Verification items for the finished model (mm, model axes). A direction names the side the tool comes from. Coordinates: 2 decimals unless noted, no trailing zeros. Write each loop counter-clockwise with the first axis right and the second up, starting at its lowest first coordinate (ties: lowest second). Pieces come first, ordered by that corner, then holes. Notation, with made-up numbers: (55, -32) -> (69, -32) arc R14 cw to (69, -20) -> close; hole circle Ø11 at (41.5, 56.25). An arc over 180 degrees is marked (long way). Write each question's results on one line, items separated by ' | '. Start each with the question number.
from build123d import *

# Parameters (mm, degrees)
F0_W     = 121.512517333
F0_H     = 63.0381852388
F1_DEPTH = 2.54
F3_R     = 10.4902
F2_R     = 10.4902
F2_R_2   = 10.4891359602
F4_DEPTH = 5.08
F5_W     = 24.793356657
F5_H     = 18.3770691669
F6_DEPTH = 4.4237


with BuildPart() as f1:
    # F0 (on Top) → F1 (new body)
    with BuildSketch(Plane.XY):
        Rectangle(F0_W, F0_H)
    extrude(amount=F1_DEPTH)

    # F3 (on face) + F2 (on face) → F4 (join)
    with BuildSketch(Plane(origin=(0, 31.5190926194, 0), x_dir=(-1, 0, 0), z_dir=(0, 1, 0))):
        with Locations((-47.3014861345, 0)):
            Circle(F3_R)
        with Locations((39.0958227217, 0)):
            Circle(F3_R)
    with BuildSketch(Plane.XZ.offset(31.5190926194)):
        with Locations((-42.2156155109, 0)):
            Circle(F2_R)
        with Locations((44.4975420833, 0)):
            Circle(F2_R_2)
    extrude(amount=F4_DEPTH, dir=(0, 1, 0))

    # F5 (on face) → F6 (join)
    with BuildSketch(Plane.YZ.offset(60.7562586665)):
        with Locations((-0.8818171918, 11.7285345834)):
            Rectangle(F5_W, F5_H)
    extrude(amount=-F6_DEPTH)


solid = f1.part
1. Material ranges on probe 1 along Y at (x, z) = (-40, -9); probe 2 along Z at (x, y) = (14.5, 8); probe 3 along Y at (x, z) = (28, 1.5), recorded low to high. Write a range as from..to.
2. Sectioned sample at B-B on z = -8. Record the cut outline in (x, y), plus the area to 3 significant figures.
3. Depth check by flat-ended pin: pin 1 Ø3 at (x, y) = (-18.5, -15) entering from -Z; pin 2 Ø5.5 at (y, z) = (2, 11.5) entering from -X; pin 3 Ø3.5 at (x, z) = (59.5, 15) entering from -Y. Enter the tip coordinate at first touch or a pass-through.
4. Mould release check, pull along Y, two halves, no side actions. Record for faces 5 (the flat face through (-39, 36.599, 0)), 6 (the cylindrical face through (-42.446, -29.015, -10.488)), 7 (the flat face through (47, 31.519, -4)): +Y half, -Y half, draft (parallel to the pull), parting line (faces both ways), or undercut.
5. Sectioned sample at D-D on z = 17. Record the cut outline in (x, y), plus the area to 3 significant figures.
6. Sectioned sample at C-C on x = -45.5. Record the cut outline in (y, z).
7. Tool access check on faces 1 (the cylindrical face through (-42.02, -29.01, 10.49)), 2 (the cylindrical face through (-28.616, 34.024, 0.461)), 3 (the flat face through (-39, 31.519, -4)), 4 (the flat face through (-42, -26.439, 6)). Record the directions out of +Z, -Z, +X, -X, +Y, -Y that give a thin tool (end or side, any length) a straight path to the whole face; none if there is none.
8. Sectioned sample at A-A on y = -3. Record the cut outline in (x, z), plus the area to 3 significant figures.
Computed values:
1) probe 1: y = -31.52..-26.44, 31.52..36.6 | probe 2: z = 0..2.54 | probe 3: y = -31.52..31.52
2) outline: (-49, -31.52) -> (-35.43, -31.52) -> (-35.43, -26.44) -> (-49, -26.44) -> close; (-45.88, 31.52) -> (-32.31, 31.52) -> (-32.31, 36.6) -> (-45.88, 36.6) -> close; (37.71, -31.52) -> (51.28, -31.52) -> (51.28, -26.44) -> (37.71, -26.44) -> close; (40.52, 31.52) -> (54.09, 31.52) -> (54.09, 36.6) -> (40.52, 36.6) -> close | area: 276 mm^2
3) pin 1: stops at z = 0 | pin 2: stops at x = 56.33 | pin 3: stops at y = -13.28
4) face 5: +Y half | face 6: draft | face 7: undercut
5) outline: (56.33, -13.28) -> (60.76, -13.28) -> (60.76, 11.51) -> (56.33, 11.51) -> close | area: 110 mm^2
6) outline: (-31.52, -9.96) -> (-26.44, -9.96) -> (-26.44, 0) -> (31.52, 0) -> (31.52, -8.31) -> (36.6, -8.31) -> (36.6, 8.31) -> (31.52, 8.31) -> (31.52, 2.54) -> (-26.44, 2.54) -> (-26.44, 9.96) -> (-31.52, 9.96) -> close
7) face 1: +Z, -Y | face 2: +Y | face 3: -Z, +X, -X | face 4: +Z, +X, -X
8) outline: (-60.76, 0) -> (60.76, 0) -> (60.76, 20.92) -> (56.33, 20.92) -> (56.33, 2.54) -> (-60.76, 2.54) -> close | area: 390 mm^2
